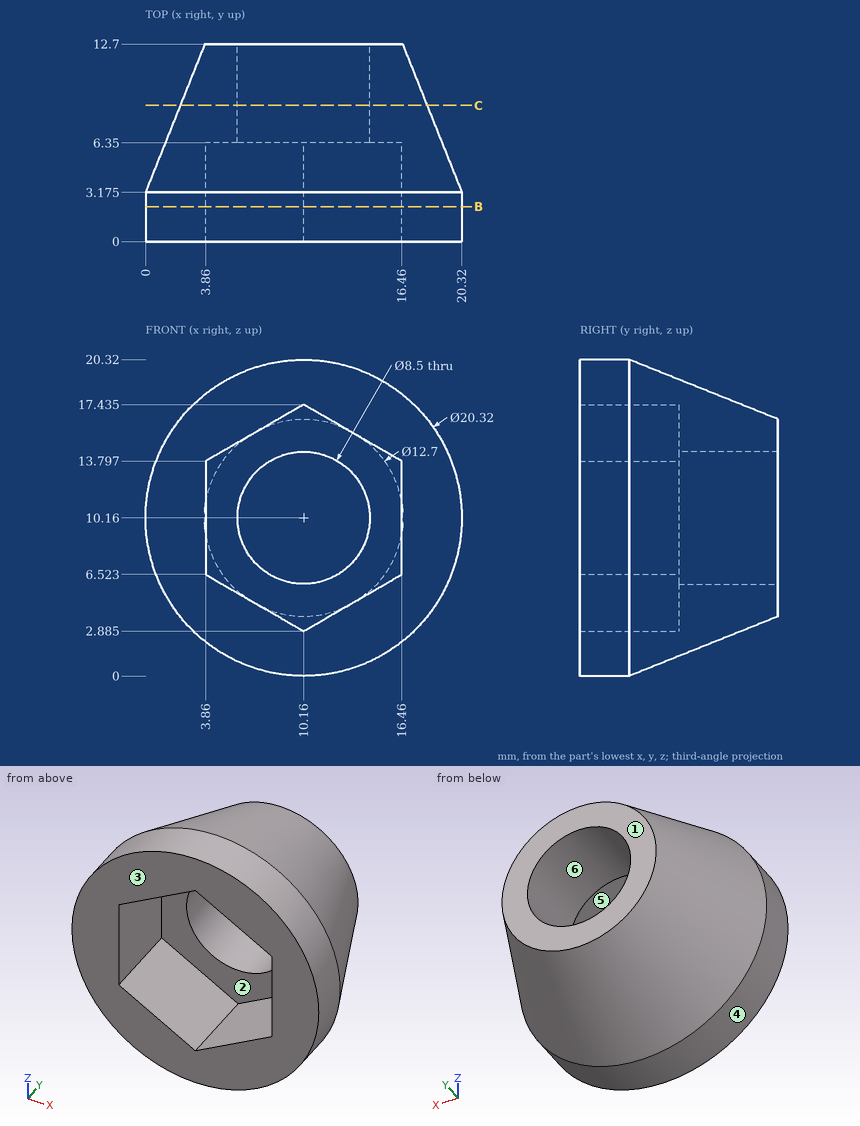
Geometry check sheet. Reference: drawing and pictorial views, mm from the part's lowest x, y, z. A direction names the side the tool comes from. Round coordinates to 2 decimals unless told otherwise and drop trailing zeros. Order: outer loops, then holes, each group sorted by start corner. A loop starts at its lowest first (then second) coordinate and runs counter-clockwise, first axis right, second up. Notation, with made-up numbers: M 50,73.5 L 79,73.5 A21 cw 79,89.5 Z; hole C 12,79.5 d9. An arc over 180 degrees is marked long. One line per item, written item: value. Start each with the question number.
1. Section check C-C on y = 8.75. Enter the section's corners in (x, z), and give its area (3 significant figures).
2. Gauge pin test, flat ends, axial feed: P1, Ø1.5, axis at y = 8, z = 16, coming from the +X side; P2, Ø1.5, axis at x = 9, y = 6.5, coming from the +Z side; P3, Ø1.9, axis at y = 4.5, z = 8.5, coming from the -X side. Record the tip position at first contact, or that the pin passes through.
3. Access from +Z, -Z, +X, -X, +Y, -Y to the whole of each face (thin tool, end or side, straight path). Record for the marked faces 1 and 2.
4. Release check for a two-part mould opening along X. For the marked faces 3, 4, 5 and 6 record: released by +X, released by -X, zero draft, split by the parting line, or undercut.
5. Scan lines: line 1 along X through (y, z) = (8, 10.16); line 2 along X through (y, z) = (3, 5.5) (1 decimal); line 3 along Z through (x, y) = (12.25, 9.5). Record each from-to range of solid material in increasing order.
6. Section check B-B on y = 2.25. Enter the section's corners in (x, z) (1 decimal).
Results found:
1. outline: C 10.16,10.16 d15.86; hole C 10.16,10.16 d8.5
1. area: 141 mm^2
2. P1: x = 16.74
2. P2: z = 19.23
2. P3: x = 0.26
3. face 1: +Z, -Z, +X, -X, +Y
3. face 2: -Y
4. face 3: zero draft
4. face 4: split by the parting line
4. face 5: undercut
4. face 6: undercut
5. line 1: 1.93 to 5.91, 14.41 to 18.39
5. line 2: 1.1 to 5.6, 14.7 to 19.2
5. line 3: 2.82 to 6.46, 13.86 to 17.5
6. outline: C 10.2,10.2 d20.3; hole M 3.9,6.5 L 10.2,2.9 L 16.5,6.5 L 16.5,13.8 L 10.2,17.4 L 3.9,13.8 Z
